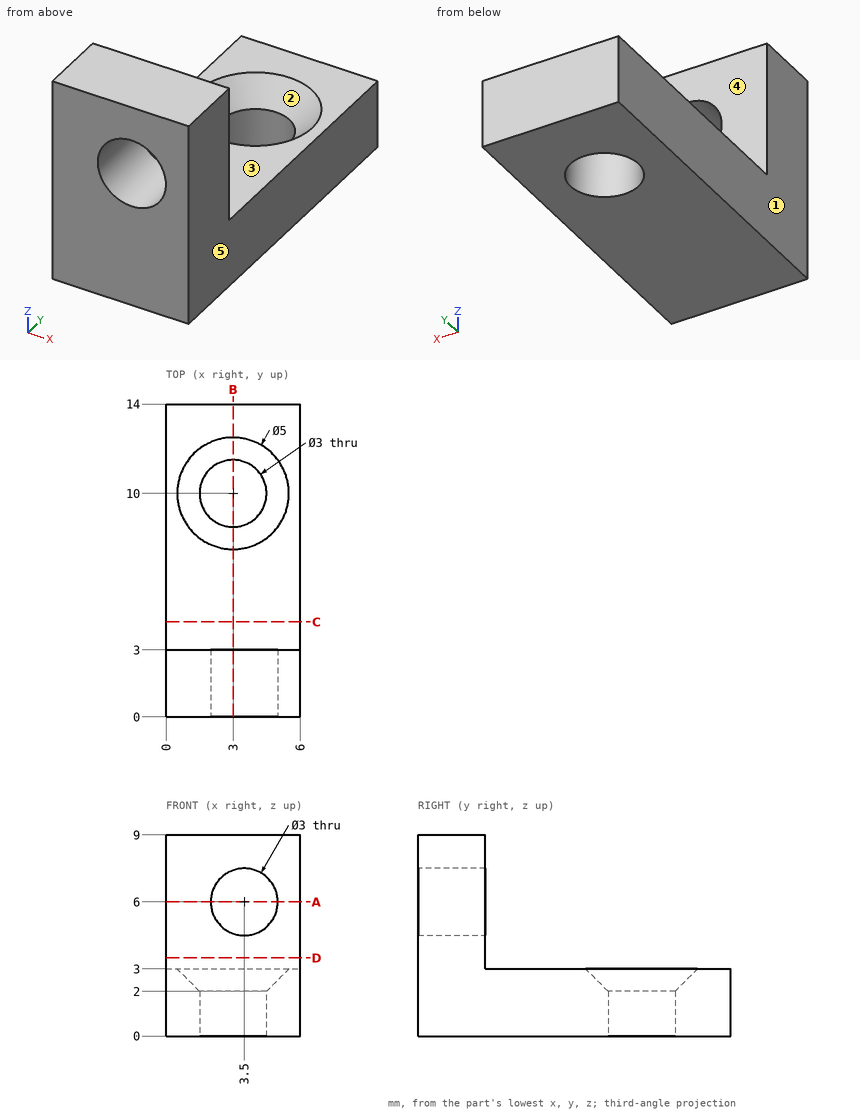
Answer from the drawing. Dimensions are ordinates in mm from the lowest x, y and z of the part. A direction names the side the tool comes from. Coordinates: 2 decimals unless noted, no trailing zeros. Write each loop counter-clockwise with the first axis right and the second up, starting at its lowest first coordinate (ties: lowest second). Pieces come first, ordered by that corner, then holes. Notation, with made-up numbers: M 6,-35 L 50,-35 A6 cw 50,-25 Z; hole C 12.25,-16.75 d6. An arc over 180 degrees is marked long. Use a Markdown table: item, result.
Q1. Determine the mould class of the marked faces 1, 2 and 3 for opening direction X: released by +X, released by -X, zero draft, split by the parting line, or undercut.
Answer block:
| item | result |
|---|---|
| face 1 | released by -X |
| face 2 | undercut |
| face 3 | zero draft |
Q2. The part is cut by section A-A, the plane z = 6. Write down the section's boundary in (x, y).
Answer block:
| item | result |
|---|---|
| outline | M 0,0 L 2,0 L 2,3 L 0,3 Z; M 5,0 L 6,0 L 6,3 L 5,3 Z |
Q3. Each of these flat-tipped pins is pushed along its axis until it touches: pin 1 Ø3.5 at (x, z) = (3.5, 6) entering from -Y; pin 2 Ø2 at (x, y) = (3.5, 6) entering from +Z. Where does it stop, or does it pass through?
Answer block:
| item | result |
|---|---|
| pin 1 | stops at y = 0 |
| pin 2 | stops at z = 3 |
Q4. The part is cut by section C-C, the plane y = 4.25. Write down the section's boundary in (x, z), then the cut area to 3 significant figures.
Answer block:
| item | result |
|---|---|
| outline | M 0,0 L 6,0 L 6,3 L 0,3 Z |
| area | 18.0 mm2 |
Q5. Straight lines are drawn through the part: L1, parallel to Y at x = 3, z = 0.5; L2, parallel to X at y = 0.7, z = 6; L3, parallel to Z at x = 5.55, y = 13. For each, find the intervals that lie inside material, in ascending order. Write a range as [from, to].
Answer block:
| item | result |
|---|---|
| L1 | y = [0, 8.5], [11.5, 14] |
| L2 | x = [0, 2], [5, 6] |
| L3 | z = [0, 3] |
Q6. Which of the six approach directions +Z, -Z, +X, -X, +Y, -Y give full straight-line access (tool end or side, diameter ignored) to the marked faces 4 and 5?
Answer block:
| item | result |
|---|---|
| face 4 | +Z, +X, -X, +Y |
| face 5 | +Z, -Z, +X, +Y, -Y |
Q7. The part is cut by section B-B, the plane x = 3. Write down the section's boundary in (y, z), then the cut area to 3 significant figures.
Answer block:
| item | result |
|---|---|
| outline | M 0,0 L 8.5,0 L 8.5,2 L 7.5,3 L 3,3 L 3,4.59 L 0,4.59 Z; M 0,7.41 L 3,7.41 L 3,9 L 0,9 Z; M 11.5,0 L 14,0 L 14,3 L 12.5,3 L 11.5,2 Z |
| area | 41.5 mm2 |
